CAD build for the part. Positions are in the model's coordinates, mm. Face numbers are marked on the shaded views. A direction names the side the tool comes from. Coordinates: 2 decimals unless noted, no trailing zeros. Order: outer loops, then holes, each group sorted by start corner. A loop starts at its lowest first (then second) coordinate and runs counter-clockwise, first axis right, second up. Notation, with made-up numbers: (-27.5, -31.75) - (-17.5, -31.75) arc R26 cw to (-17.5, -14.75) - close; hole circle Ø9 at (40.5, 15). An arc over 180 degrees is marked (long way). Write each question's results on one line, items separated by ' | '. Start each with the question number.
Q1. Band-saw the part on B-B, the plane x = 43. Write the cut outline in (y, z).
Q2. Band-saw the part on C-C, the plane y = -62.5. Write the cut outline in (x, z), then the cut area to 3 significant figures.
Q3. Wall check: probe 1 along Z at (x, y) = (10, 70); probe 2 along Y at (x, z) = (30, 2); probe 3 along Y at (x, z) = (3, -65.5). Give the ranges that are in metal, low to high.
Q4. Pull direction Z, two halves, no side cores. Call the marked faces 4, 5, 6 and 7: released by +Z, released by -Z, zero draft, split by the parting line, or undercut.
Q5. Which spindle directions (+Z, -Z, +X, -X, +Y, -Y) get a long thin tool onto all of the face, cutting with end or side? Do the marked faces 1, 2 and 3. Say none if no direction does.
Q6. Band-saw the part on A-A, the plane z = -33.5. Write the cut outline in (x, y).
Q7. Pin check, flat tips, straight feed: P1, Ø22, axis at x = 1.61, z = -40, coming from the +Y side; P2, Ø11.5, axis at y = 36, z = -12.5, coming from the +X side; P3, Ø1.5, axis at x = 19, z = -17.5, coming from the -Y side. Stop position of each tip, or through.
Q8. Band-saw the part on D-D, the plane x = 31.5. Write the cut outline in (y, z).
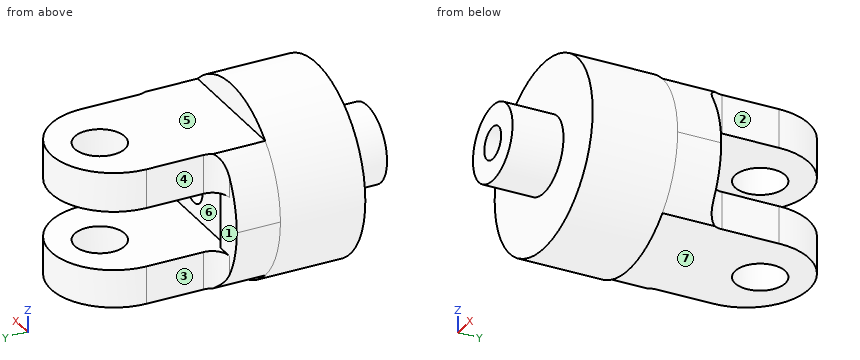
```python
from build123d import *

# Parameters (mm, degrees)
BOSS_EXTRUDE1_DEPTH = 80
SKETCH2_R           = 14.752980174
CUT_EXTRUDE1_DEPTH  = 80
SKETCH3_R           = 55.298116799
BOSS_EXTRUDE2_DEPTH = 50
SKETCH4_R           = 22.325866005
BOSS_EXTRUDE3_DEPTH = 30
CUT_EXTRUDE2_DEPTH  = 30
CUT_EXTRUDE3_DEPTH  = 30
CUT_EXTRUDE4_DEPTH  = 30
CUT_EXTRUDE5_DEPTH  = 30
SKETCH11_W          = 73.883790911
SKETCH11_H          = 34.739224631
CUT_EXTRUDE9_DEPTH  = 110
FILLET1_R           = 10
SKETCH12_R          = 9.507720781
CUT_EXTRUDE10_DEPTH = 110


with BuildPart() as part:
    # Sketch1 → Boss-Extrude1 (new body)
    with BuildSketch(Plane.XY):
        with BuildLine():
            Line((-53.691947432, 3.671244269), (-35.335726088, 3.671244269))
            Line((-35.335726088, 3.671244269), (-35.335726088, 47.267269961))
            ThreePointArc((-35.335726088, 47.267269961), (1.606169368, 84.209165417), (38.548064823, 47.267269961))
            Line((38.548064823, 47.267269961), (38.548064823, 3.671244269))
            Line((38.548064823, 3.671244269), (56.904286167, 3.671244269))
            Line((56.904286167, 3.671244269), (56.904286167, -22.027465613))
            Line((56.904286167, -22.027465613), (-53.691947432, -22.027465613))
            Line((-53.691947432, -22.027465613), (-53.691947432, 3.671244269))
        make_face()
    extrude(amount=-BOSS_EXTRUDE1_DEPTH)

    # Sketch2 → Cut-Extrude1 (cut)
    with BuildSketch(Plane.XY):
        with Locations((1.606169368, 55.478429373)):
            Circle(SKETCH2_R)
    extrude(amount=-CUT_EXTRUDE1_DEPTH, mode=Mode.SUBTRACT)

    # Sketch3 → Boss-Extrude2 (add)
    with BuildSketch(Plane.XZ.offset(22.027465613)):
        with Locations((1.606169368, -40)):
            Circle(SKETCH3_R)
    extrude(amount=BOSS_EXTRUDE2_DEPTH)

    # Sketch4 → Boss-Extrude3 (add)
    with BuildSketch(Plane.XZ.offset(72.027465613)):
        with Locations((1.606169368, -40)):
            Circle(SKETCH4_R)
    extrude(amount=BOSS_EXTRUDE3_DEPTH)

    # Sketch5 → Cut-Extrude2 (cut)
    with BuildSketch(Plane.XZ.offset(22.027465613)):
        with BuildLine():
            Line((-36.57604798, 0), (-53.691947432, 0))
            Line((-53.691947432, 0), (-53.691947432, -40))
            ThreePointArc((-53.691947432, -40), (-49.233217116, -18.245954318), (-36.57604798, 0))
        make_face()
    extrude(amount=-CUT_EXTRUDE2_DEPTH, mode=Mode.SUBTRACT)

    # Sketch6 → Cut-Extrude3 (cut)
    with BuildSketch(Plane.XZ.offset(22.027465613)):
        with BuildLine():
            Line((-36.57604798, -80), (-53.691947432, -80))
            Line((-53.691947432, -80), (-53.691947432, -40))
            ThreePointArc((-53.691947432, -40), (-49.233217116, -61.754045682), (-36.57604798, -80))
        make_face()
    extrude(amount=-CUT_EXTRUDE3_DEPTH, mode=Mode.SUBTRACT)

    # Sketch7 → Cut-Extrude4 (cut)
    with BuildSketch(Plane.XZ.offset(22.027465613)):
        with BuildLine():
            Line((56.904286167, -40), (56.904286167, 0))
            Line((56.904286167, 0), (39.788386715, 0))
            ThreePointArc((39.788386715, 0), (52.445555851, -18.245954318), (56.904286167, -40))
        make_face()
    extrude(amount=-CUT_EXTRUDE4_DEPTH, mode=Mode.SUBTRACT)

    # Sketch8 → Cut-Extrude5 (cut)
    with BuildSketch(Plane.XZ.offset(22.027465613)):
        with BuildLine():
            Line((39.788386715, -80), (56.904286167, -80))
            Line((56.904286167, -80), (56.904286167, -40))
            ThreePointArc((56.904286167, -40), (52.445555851, -61.754045682), (39.788386715, -80))
        make_face()
    extrude(amount=-CUT_EXTRUDE5_DEPTH, mode=Mode.SUBTRACT)

    # Sketch11 → Cut-Extrude9 (cut)
    with BuildSketch(Plane(origin=(0, 0, 0), x_dir=(1, 0, 0), z_dir=(0, 1, 0))):
        with Locations((1.606169368, 40.391795767)):
            Rectangle(SKETCH11_W, SKETCH11_H)
    extrude(amount=CUT_EXTRUDE9_DEPTH, mode=Mode.SUBTRACT)

    # Fillet1
    fillet1_edges = [part.edges().sort_by_distance(p)[0] for p in [
        (-35.335726088, 3.671244269, -68.880704041),
        (38.548064823, 3.671244269, -68.880704041),
        (38.548064823, 3.671244269, -11.511091725),
        (-35.335726088, 3.671244269, -11.511091725),
    ]]
    fillet(fillet1_edges, radius=FILLET1_R)

    # Sketch12 → Cut-Extrude10 (cut)
    with BuildSketch(Plane.XZ.offset(102.027465613)):
        with Locations((1.606169368, -40)):
            Circle(SKETCH12_R)
    extrude(amount=-CUT_EXTRUDE10_DEPTH, mode=Mode.SUBTRACT)


solid = part.part
```
Results below:
1) outline: (-72.03, -76.67) - (5.35, -76.67) - (5.35, -57.76) - (3.67, -57.76) - (3.67, -23.02) - (5.35, -23.02) - (5.35, -3.33) - (-72.03, -3.33) - close
2) outline: circle Ø110.6 at (1.61, -40); hole circle Ø19.02 at (1.61, -40) | area: 9,320 mm²
3) probe 1: z = -80 to -57.76, -23.02 to 0 | probe 2: y = -72.03 to -22.03 | probe 3: y = -72.03 to 40.79, 70.17 to 84.18
4) face 4: zero draft | face 5: released by +Z | face 6: undercut | face 7: released by -Z
5) face 1: -X, +Y | face 2: +Z, -Z, +X, +Y | face 3: +Z, -Z, -X, +Y
6) outline: (-53.31, -72.03) - (-19.75, -72.03) - (-19.75, -102.03) - (-5.33, -102.03) - (-5.33, 0) - (-35.34, 0) - (-35.34, 3.67) - (-53.31, 3.67) - close; (8.54, -102.03) - (22.96, -102.03) - (22.96, -72.03) - (56.52, -72.03) - (56.52, 3.67) - (38.55, 3.67) - (38.55, 0) - (8.54, 0) - close
7) P1: stops at y = 0 | P2: stops at x = 38.55 | P3: stops at y = -72.03
8) outline: (-72.03, -86.52) - (-22.03, -86.52) - (-22.03, -80) - (68.97, -80) - (68.97, -57.76) - (0, -57.76) - (0, -23.02) - (68.97, -23.02) - (68.97, 0) - (-22.03, 0) - (-22.03, 6.52) - (-72.03, 6.52) - close
